from build123d import *

# Parameters (mm, degrees)
F0_W     = 76.2
F0_H     = 50.8
F1_DEPTH = 25.4
F2_DEPTH = 31.75


with BuildPart() as f1:
    # F0 (on Front) → F1 (new body, symmetric)
    with BuildSketch(Plane.XZ):
        Rectangle(F0_W, F0_H)
    extrude(amount=F1_DEPTH, both=True)

    # F0 (on Front) → F2 (join, symmetric)
    with BuildSketch(Plane.XZ):
        Polygon((0, 47.397045), (-38.1, 25.4), (38.1, 25.4), align=None)
    extrude(amount=F2_DEPTH, both=True)


solid = f1.part
For this review, take the finished solid that the model builds, in its own axes (mm). A direction names the side the tool comes from. Give positions to 0.01 mm unless a question says otherwise; leave off trailing zeros. Loops run counter-clockwise (first coordinate to the right, second up) from the corner with the lowest first, then second, coordinate; pieces in that order, holes last. Notation, with made-up numbers: M -37,-25 L -8,-25 A14 cw -8,-5 Z; hole C 32.5,85.25 d9. An arc over 180 degrees is marked long. Answer as a JSON object with one key per item and string values. Group by question number.
Q1. For probe 1 along Y at (x, z) = (25, 22); probe 2 along X at (y, z) = (-11, 41.5); probe 3 along Z at (x, y) = (-3, -23) (3 decimals), list the stretches that pass through material, from the lowest coordinate up. Write a range as [from, to].
Q2. Add section C-C on z = -6. Give the boundary of the cut face in (x, y).
Q3. Add section D-D on x = 27.5. Give the boundary of the cut face in (y, z), and give its area (3 significant figures).
Q4. Insertion check: P1, Ø5, axis at x = -22.5, y = -17.5, coming from the +Z side; P2, Ø1.5, axis at x = 6, z = 3.5, coming from the +Y side; P3, Ø6, axis at x = 6, y = 2.5, coming from the +Z side (3 decimals). Each pin has a flat end and moves straight along its axis. Give the tip position at first contact, or say it passes through.
Q5. Add section A-A on y = -11.5. Give the boundary of the cut face in (x, z).
Q6. Tool access review of faces 1 (the flat face through (-1, -29, 25.4)), 2 (the flat face through (-1, 29, 25.4)), 3 (the flat face through (-1, 31.75, 34)): name each direction out of +Z, -Z, +X, -X, +Y, -Y from which nothing blocks a thin tool from reaching the whole face with its end or side.
Q7. Add section B-B on x = -14. Give the boundary of the cut face in (y, z).
Checked values:
{
 "1": {"probe 1": "[-25.4, 25.4]", "probe 2": "[-10.21, 10.21]", "probe 3": "[-25.4, 45.665]"},
 "2": {"outline": "M -38.1,-25.4 L 38.1,-25.4 L 38.1,25.4 L -38.1,25.4 Z"},
 "3": {"outline": "M -31.75,25.4 L -25.4,25.4 L -25.4,-25.4 L 25.4,-25.4 L 25.4,25.4 L 31.75,25.4 L 31.75,31.52 L -31.75,31.52 Z", "area": "2,970 mm²"},
 "4": {"P1": "z = 35.85", "P2": "y = 25.4", "P3": "z = 45.665"},
 "5": {"outline": "M -38.1,-25.4 L 38.1,-25.4 L 38.1,25.4 L 0,47.4 L -38.1,25.4 Z"},
 "6": {"face 1": "-Z, +X, -X, -Y", "face 2": "-Z, +X, -X, +Y", "face 3": "+Z, -Z, +X, -X, +Y"},
 "7": {"outline": "M -31.75,25.4 L -25.4,25.4 L -25.4,-25.4 L 25.4,-25.4 L 25.4,25.4 L 31.75,25.4 L 31.75,39.31 L -31.75,39.31 Z"}
}
